Here's how the part is built. I have some questions about the finished solid (model axes, mm). A direction names the side the tool comes from. Give positions to 0.01 mm unless a question says otherwise; leave off trailing zeros. Write each loop counter-clockwise with the first axis right and the second up, starting at its lowest first coordinate (ties: lowest second). Pieces come first, ordered by that corner, then holes. Notation, with made-up numbers: (-12, -0.5) - (12, -0.5) arc R16 ccw to (12, 16.5) - close; hole circle Ø1 at (-10, 41). An arc over 180 degrees is marked (long way). Use a Markdown table: item, result.
```python
from build123d import *

# Parameters (mm, degrees)
SKETCH1_W           = 100
SKETCH1_H           = 100
BOSS_EXTRUDE1_DEPTH = 180
SKETCH2_R           = 34.257790197
BOSS_EXTRUDE2_DEPTH = 350
SKETCH3_W           = 152.006357392
SKETCH3_H           = 282.452416457
CUT_EXTRUDE2_DEPTH  = 400
CUT_EXTRUDE3_DEPTH  = 400
CUT_EXTRUDE4_DEPTH  = 400
CUT_EXTRUDE5_DEPTH  = 400
SKETCH7_W           = 160.159381639
SKETCH7_H           = 147.362276113
CUT_EXTRUDE6_DEPTH  = 400
SKETCH8_W           = 147.310744502
SKETCH8_H           = 162.038906966
CUT_EXTRUDE7_DEPTH  = 400
SKETCH9_R           = 31.847293423
CUT_EXTRUDE8_DEPTH  = 400
SKETCH10_W          = 140.220962397
SKETCH10_H          = 212.033531124
CUT_EXTRUDE9_DEPTH  = 400
SKETCH11_R          = 13.603137886
CUT_EXTRUDE11_DEPTH = 15
SKETCH12_R          = 12.495422516
BOSS_EXTRUDE3_DEPTH = 15
SKETCH13_R          = 1.594865099
BOSS_EXTRUDE4_DEPTH = 4
SKETCH14_W          = 100.74862993
SKETCH14_H          = 110.555003588
CUT_EXTRUDE13_DEPTH = 400


with BuildPart() as part:
    # Sketch1 → Boss-Extrude1 (new body)
    with BuildSketch(Plane(origin=(0, 0, 0), x_dir=(1, 0, 0), z_dir=(0, 1, 0))):
        with Locations((-50, 50)):
            Rectangle(SKETCH1_W, SKETCH1_H)
    extrude(amount=BOSS_EXTRUDE1_DEPTH)

    # Sketch2 → Boss-Extrude2 (add, symmetric)
    with BuildSketch(Plane(origin=(0, 180, 0), x_dir=(1, 0, 0), z_dir=(0, 1, 0))):
        with Locations(Location((-51.377291833, 49.076536384, 0), (0, 0, 270))):
            Circle(SKETCH2_R)
    extrude(amount=BOSS_EXTRUDE2_DEPTH, both=True)

    # Sketch3 → Cut-Extrude2 (cut)
    with BuildSketch(Plane(origin=(0, 0, 0), x_dir=(0, 0, -1), z_dir=(1, 0, 0))):
        with Locations((57.419900112, 502.274302507)):
            Rectangle(SKETCH3_W, SKETCH3_H)
    extrude(amount=-CUT_EXTRUDE2_DEPTH, mode=Mode.SUBTRACT)

    # Sketch4 → Cut-Extrude3 (cut)
    with BuildSketch(Plane(origin=(0, 0, 0), x_dir=(0, 0, -1), z_dir=(1, 0, 0))):
        Polygon((12.981970869, 0), (-8.994244796, 25.828096003), (-18.564506014, -15.259465835), align=None)
        Polygon((85.072517936, -1.448103984), (109.237639161, 19.113145112), (115.920034239, -3.267382694), align=None)
        Polygon((12.981970869, 180), (-8.994244796, 148.537596011), (-15.418178585, 193.219274892), align=None)
        Polygon((85.072517936, 181.854312784), (103.841225373, 159.795920888), (106.132549481, 198.647393934), align=None)
    extrude(amount=-CUT_EXTRUDE3_DEPTH, mode=Mode.SUBTRACT)

    # Sketch5 → Cut-Extrude4 (cut)
    with BuildSketch(Plane.XY):
        Polygon((-85.623287335, 0), (-106.370377984, 21.426392531), (-122.288861874, 3.209259887), (-93.526345261, -19.884701759), align=None)
        Polygon((-15.694988751, 0), (0, 15.257385304), (12.122677088, 15.257385304), (10.563067769, -19.884701759), align=None)
        Polygon((-87.166490339, 180.248071029), (-106.370377984, 151.29108453), (-117.705469457, 200.501115102), align=None)
        Polygon((-15.694988751, 180.248071029), (7.833767065, 153.279557508), (0, 193.941208308), align=None)
    extrude(amount=-CUT_EXTRUDE4_DEPTH, mode=Mode.SUBTRACT)

    # Sketch6 → Cut-Extrude5 (cut)
    with BuildSketch(Plane(origin=(0, 180, 0), x_dir=(1, 0, 0), z_dir=(0, 1, 0))):
        Polygon((-112.386997555, 28.400400964), (-64.261264503, -10.212759359), (-84.406366528, -15.51192827), (-124.649689542, -15.51192827), align=None)
        Polygon((-97.065537028, 135.861756084), (-119.37552445, 77.792688888), (-118.043343626, 64.347606737), (-66.428694172, 110.575168787), align=None)
        Polygon((-24.69640689, -21.815840769), (11.092108798, -8.97361337), (17.428316417, 32.393768119), (-38.531576846, -11.139157378), align=None)
        Polygon((-17.445484601, 140.804394854), (35.417473102, 107.262520599), (9.305452855, 72.996438725), (-31.724385352, 103.625272537), align=None)
    extrude(amount=-CUT_EXTRUDE5_DEPTH, mode=Mode.SUBTRACT)

    # Sketch7 → Cut-Extrude6 (cut)
    with BuildSketch(Plane.XY):
        with Locations((-66.123258915, -136.36252694)):
            Rectangle(SKETCH7_W, SKETCH7_H)
    extrude(amount=-CUT_EXTRUDE6_DEPTH, mode=Mode.SUBTRACT)

    # Sketch8 → Cut-Extrude7 (cut)
    with BuildSketch(Plane.XY):
        with Locations((-53.541153336, 332.448287589)):
            Rectangle(SKETCH8_W, SKETCH8_H)
    extrude(amount=-CUT_EXTRUDE7_DEPTH, mode=Mode.SUBTRACT)

    # Sketch9 → Cut-Extrude8 (cut)
    with BuildSketch(Plane(origin=(0, 251.428834106, 0), x_dir=(1, 0, 0), z_dir=(0, 1, 0))):
        with Locations(Location((-50.808993157, 49.032036374, 0), (0, 0, 270))):
            Circle(SKETCH9_R)
    extrude(amount=-CUT_EXTRUDE8_DEPTH, mode=Mode.SUBTRACT)

    # Sketch10 → Cut-Extrude9 (cut)
    with BuildSketch(Plane.ZY.offset(100)):
        with Locations((14.299084536, 180.100625535)):
            Rectangle(SKETCH10_W, SKETCH10_H)
    extrude(amount=-CUT_EXTRUDE9_DEPTH, mode=Mode.SUBTRACT)

    # Sketch11 → Cut-Extrude11 (cut)
    with BuildSketch(Plane.ZY.offset(100)):
        with Locations((-50.413251954, 76.264646142)):
            Circle(SKETCH11_R)
    extrude(amount=-CUT_EXTRUDE11_DEPTH, mode=Mode.SUBTRACT)

    # Sketch12 → Boss-Extrude3 (add)
    with BuildSketch(Plane.ZY.offset(85)):
        with Locations(Location((-50.658800768, 76.222522328, 0), (0, 0, 114.353089558))):
            Circle(SKETCH12_R)
    extrude(amount=BOSS_EXTRUDE3_DEPTH)

    # Sketch13 → Boss-Extrude4 (add)
    with BuildSketch(Plane(origin=(-85, 0, 0), x_dir=(0, 0, -1), z_dir=(1, 0, 0))):
        with Locations(Location((49.945205578, 75.944780088, 0), (0, 0, 180))):
            Circle(SKETCH13_R)
    extrude(amount=BOSS_EXTRUDE4_DEPTH)

    # Sketch14 → Cut-Extrude13 (cut)
    with BuildSketch(Plane.ZY.offset(100)):
        with Locations((-65.350029467, 250.603414818)):
            Rectangle(SKETCH14_W, SKETCH14_H)
    extrude(amount=-CUT_EXTRUDE13_DEPTH, mode=Mode.SUBTRACT)


solid = part.part
```
Item 1: For faces 1 (the cylindrical face through (-50.72, 187.77, -83.33)), 2 (the cylindrical face through (-92.395, 64.623, -46.012)), 3 (the flat face through (-13.246, 90.863, -89.831)), which set-ups out of +Z, -Z, +X, -X, +Y, -Y let a thin tool reach every point of the face, with its end or its side?
Values:
| item | result |
|---|---|
| face 1 | -Z, +Y |
| face 2 | -X |
| face 3 | -Z, +X, +Y, -Y |
Item 2: If we section it at B-B, the plane x = -39.5: Write out the boundary of the cut face in (y, z).
Values:
| item | result |
|---|---|
| outline | (-62.68, -81.21) - (0, -81.21) - (0, -86.77) - (11.25, -100) - (164.31, -100) - (180, -86.65) - (180, -81.21) - (195.33, -81.21) - (195.33, -78.8) - (-62.68, -78.8) - close; (-62.68, -19.26) - (74.08, -19.26) - (74.08, 0) - (15.26, 0) - (0, -12.98) - (0, -16.94) - (-62.68, -16.94) - close |
Item 3: If we section it at A-A, the plane z = -44: Write out the boundary of the cut face in (x, y), plus the area to 3 significant figures.
Values:
| item | result |
|---|---|
| outline | (-100, 14.85) - (-85.62, 0) - (-85.26, 0) - (-85.26, -62.68) - (-82.26, -62.68) - (-82.26, 74.08) - (-85, 74.08) - (-85, 86.8) - (-100, 86.8) - (-100, 65.65) - (-85, 65.65) - (-85, 64.27) - (-100, 64.27) - close; (-19.36, -62.68) - (-17.5, -62.68) - (-17.5, 0) - (-15.69, 0) - (0, 15.26) - (0, 74.08) - (-19.36, 74.08) - close |
| area | 3,000 mm2 |
Item 4: Thinking about a two-plate mould opening in X: for faces 4 (the cylindrical face through (-70.188, 39.461, -74.305)), 5 (the cylindrical face through (-92.6, 65.78, -59.08)), 6 (the flat face through (-85, 65, -57)), 7 (the cylindrical face through (-84.82, -30.9, -56.5)), which applies, +X half, -X half, draft (parallel to the pull), parting line (faces both ways), or undercut?
Values:
| item | result |
|---|---|
| face 4 | undercut |
| face 5 | draft |
| face 6 | -X half |
| face 7 | parting line |
Item 5: I need wall thicknesses on line 1 along X through (y, z) = (76.5, -45); line 2 along Y through (x, z) = (-35, -16.5); line 3 along X through (y, z) = (-41, -70). Which ranges of each line are inside material? Lowest first, please. Write a range as [from, to].
Values:
| item | result |
|---|---|
| line 1 | x = [-100, -85] |
| line 2 | y = [0, 74.08] |
| line 3 | x = [-78.5, -74.78], [-26.84, -24.25] |
Item 6: If we section it at C-C, the plane y = 145: Write out the boundary of the cut face in (x, z).
Values:
| item | result |
|---|---|
| outline | (-100, -80.51) - (-78.24, -100) - (-26.87, -100) - (0, -79.94) - (0, -55.81) - (-19.69, -55.81) arc R31.85 cw to (-81.93, -55.81) - (-100, -55.81) - close |
Item 7: Will these pins go through, and if not, where does the flat tip stop? pin 1 Ø2 at (x, y) = (-85, 48) entering from +Z; pin 2 Ø1 at (x, y) = (-85.5, 24.5) entering from +Z; pin 3 Ø9 at (x, y) = (-89, 161.5) entering from +Z.
Values:
| item | result |
|---|---|
| pin 1 | stops at z = -5.62 |
| pin 2 | stops at z = -6.43 |
| pin 3 | stops at z = -55.81 |
Item 8: If we section it at D-D, the plane z = -74.5: Write out the boundary of the cut face in (x, y).
Values:
| item | result |
|---|---|
| outline | (-100, 14.85) - (-85.62, 0) - (-74.34, 0) - (-74.34, -62.68) - (-69.93, -62.68) - (-69.93, 195.33) - (-74.34, 195.33) - (-74.34, 180) - (-87.33, 180) - (-100, 160.9) - close; (-31.69, -62.68) - (-28.42, -62.68) - (-28.42, 0) - (-15.69, 0) - (0, 15.26) - (0, 162.26) - (-15.48, 180) - (-28.42, 180) - (-28.42, 195.33) - (-31.69, 195.33) - close |
